Answer from the drawing. Dimensions are ordinates in mm from the lowest x, y and z of the part. Give positions to 0.01 mm unless a question says otherwise; leave off trailing zeros. Write each loop counter-clockwise with the first axis right and the second up, starting at its lowest first coordinate (ties: lowest second). Pieces come first, ordered by that corner, then holes.
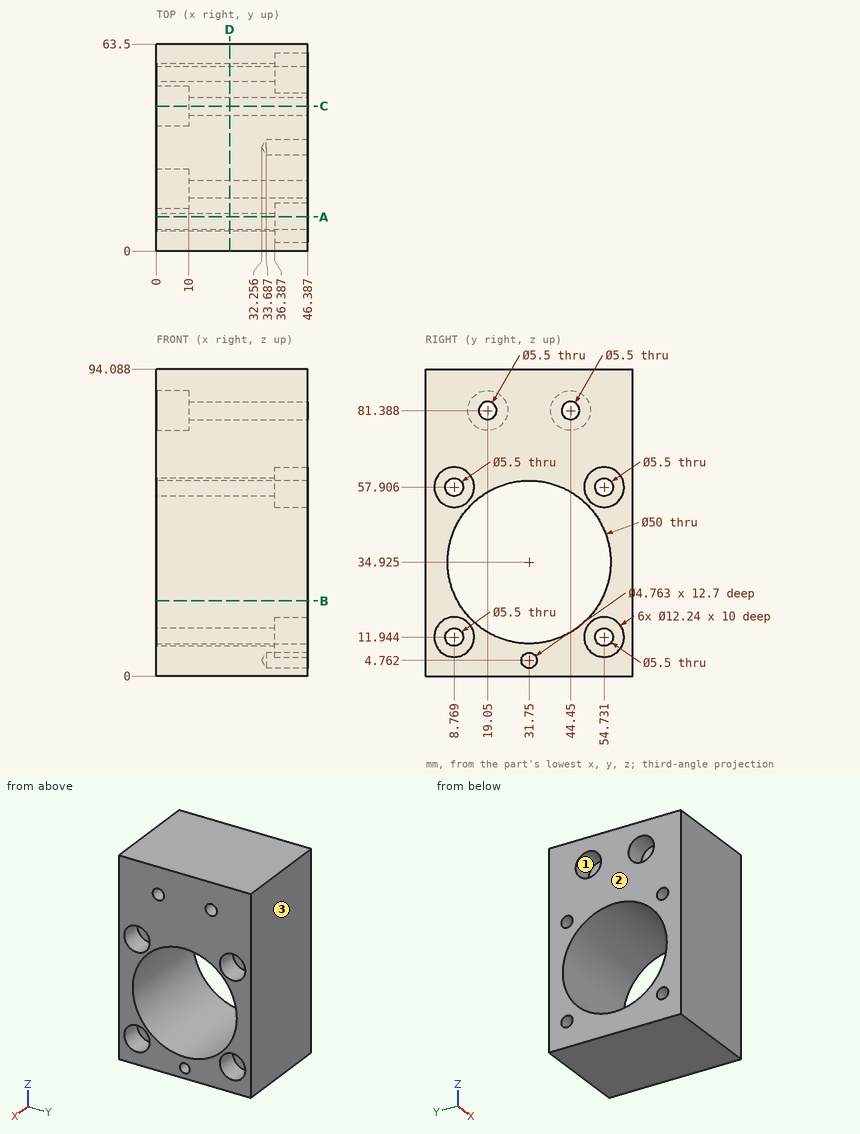
Item 1: Each of these flat-tipped pins is pushed along its axis until it touches: P1, Ø6, axis at y = 52, z = 13, coming from the +X side; P2, Ø10, axis at y = 44, z = 82, coming from the -X side. Where does it stop, or does it pass through?
Conclusion:
P1: stops at x = 36.39
P2: stops at x = 10
Item 2: A cutting plane is placed at D-D, the plane x = 22.5. Count the separate pieces of the cut face and the enclosed holes in it, plus the area to 3 significant figures.
Conclusion:
separate pieces: 1
enclosed holes: 7
area: 3,870 mm2
Item 3: Consider probe 1 along Z at (x, y) = (40, 51) (1 decimal); probe 2 along Z at (x, y) = (8, 32); probe 3 along Z at (x, y) = (7, 42) (1 decimal). Determine where each line is inside the solid, lowest interval first.
Conclusion:
probe 1: z = 0 to 7.1, 16.8 to 19, 50.9 to 53.1, 62.8 to 94.1
probe 2: z = 0 to 9.93, 59.92 to 94.09
probe 3: z = 0 to 12.1, 57.7 to 75.8, 87 to 94.1
Item 4: A cutting plane is placed at C-C, the plane y = 44.45. Give the vertices of the cut face in (x, z).
Conclusion:
outline: (0, 0) - (46.39, 0) - (46.39, 13.39) - (0, 13.39) - close; (0, 56.46) - (46.39, 56.46) - (46.39, 78.64) - (10, 78.64) - (10, 75.27) - (0, 75.27) - close; (0, 87.51) - (10, 87.51) - (10, 84.14) - (46.39, 84.14) - (46.39, 94.09) - (0, 94.09) - close
Item 5: A cutting plane is placed at B-B, the plane z = 23. Give the vertices of the cut face in (x, y), plus the area to 3 significant figures.
Conclusion:
outline: (0, 0) - (46.39, 0) - (46.39, 9.78) - (0, 9.78) - close; (0, 53.72) - (46.39, 53.72) - (46.39, 63.5) - (0, 63.5) - close
area: 907 mm2
Item 6: A cutting plane is placed at A-A, the plane y = 10.5. Give the vertices of the cut face in (x, z) (1 decimal), plus the area to 3 significant figures.
Conclusion:
outline: (0, 0) - (46.4, 0) - (46.4, 6.1) - (36.4, 6.1) - (36.4, 9.8) - (0, 9.8) - close; (0, 14.1) - (36.4, 14.1) - (36.4, 17.8) - (46.4, 17.8) - (46.4, 21.8) - (0, 21.8) - close; (0, 48.1) - (46.4, 48.1) - (46.4, 52) - (36.4, 52) - (36.4, 55.8) - (0, 55.8) - close; (0, 60) - (36.4, 60) - (36.4, 63.8) - (46.4, 63.8) - (46.4, 94.1) - (0, 94.1) - close
area: 2,600 mm2
Item 7: Determine the mould class of the marked faces 1, 2 and 3 for opening direction Y: pulls with the +Y half, pulls with the -Y half, needs draft (parallel to the pull), parting line crosses it, or undercut.
Conclusion:
face 1: undercut
face 2: needs draft
face 3: pulls with the +Y half
